The listing builds one solid part. Answer for the finished solid, in the listing's coordinates (mm). Round coordinates to 2 decimals unless told otherwise and drop trailing zeros. Loops run counter-clockwise (first coordinate to the right, second up) from the corner with the lowest first, then second, coordinate; pieces in that order, holes last. Notation, with made-up numbers: M 56,32.25 L 61,32.25 A23 ccw 61,59.25 Z; hole C -23.5,45 d3. An arc over 180 degrees is marked long. Put each result on its own line as item: value. Start each with the question number.
(1) Determine the mould class of faces 1 (the face through (0.631, 0.986, 2.003)), 2 (the face through (19.894, 1.014, -1.641)), 3 (the face through (5, 2, -7)) for opening direction X: released by +X, released by -X, zero draft, split by the parting line, or undercut.
(2) Straight lines are drawn through the part: line 1 (X direction, y = 1.1, z = 0); line 2 (X direction, y = 0.6, z = -1); line 3 (X direction, y = 1.05, z = -20). For each, find the intervals that lie inside material, in ascending order.
(3) Section A-A, the plane z = -20 is taken. Determine the outline of the cut face in (x, y).
(4) Section C-C, the plane y = 1.7 is taken. Determine the outline of the cut face in (x, z).
(5) Section D-D, the plane z = 0 is taken. Determine the outline of the cut face in (x, y).
(6) Section B-B, the plane x = 0 is taken. Determine the outline of the cut face in (y, z).
```python
from build123d import *

# Parameters (mm, degrees)
SKETCH_1_R      = 2.1
EXTRUDE_1_DEPTH = 2
FILLET_1_R      = 2


with BuildPart() as part:
    # ｽｹｯﾁ1 → ﾎﾞｽ - 押し出し1 (new body)
    with BuildSketch(Plane(origin=(0, 0, 0), x_dir=(1, 0, 0), z_dir=(0, 1, 0))):
        Polygon((-5, 25), (-5, -5), (20, -5), (20, 1.666666667), (2.5, 25), align=None)
        with Locations(Location((0, 20, 0), (0, 0, 270))):
            Circle(SKETCH_1_R, mode=Mode.SUBTRACT)
        with Locations(Location((0, 0, 0), (0, 0, 270))):
            Circle(SKETCH_1_R, mode=Mode.SUBTRACT)
        with Locations(Location((15, 0, 0), (0, 0, 270))):
            Circle(SKETCH_1_R, mode=Mode.SUBTRACT)
    extrude(amount=EXTRUDE_1_DEPTH)

    # ﾌｨﾚｯﾄ1
    fillet_1_edges = [part.edges().sort_by_distance(p)[0] for p in [
        (-5, 1, -25),
        (2.5, 1, -25),
        (20, 1, -1.666666667),
        (20, 1, 5),
        (-5, 1, 5),
    ]]
    fillet(fillet_1_edges, radius=FILLET_1_R)


solid = part.part
```
Recorded:
1. face 1: undercut
1. face 2: released by +X
1. face 3: zero draft
2. line 1: x = -5 to -2.1, 2.1 to 12.9, 17.1 to 20
2. line 2: x = -5 to -1.85, 1.85 to 13.15, 16.85 to 20
2. line 3: x = -5 to -2.1, 2.1 to 6.25
3. outline: M -5,0 L -2.1,0 L -2.1,2 L -5,2 Z; M 2.1,0 L 6.25,0 L 6.25,2 L 2.1,2 Z
4. outline: M -5,-23 A2 ccw -3,-25 L 1.5,-25 A2 ccw 3.1,-24.2 L 19.6,-2.2 A2 ccw 20,-1 L 20,3 A2 ccw 18,5 L -3,5 A2 ccw -5,3 Z; hole C 0,-20 d4.2; hole C 0,0 d4.2; hole C 15,0 d4.2
5. outline: M -5,0 L -2.1,0 L -2.1,2 L -5,2 Z; M 2.1,0 L 12.9,0 L 12.9,2 L 2.1,2 Z; M 17.1,0 L 20,0 L 20,2 L 17.1,2 Z
6. outline: M 0,-25 L 2,-25 L 2,-22.1 L 0,-22.1 Z; M 0,-17.9 L 2,-17.9 L 2,-2.1 L 0,-2.1 Z; M 0,2.1 L 2,2.1 L 2,5 L 0,5 Z
